Part model, mm, in its own coordinate system. A direction names the side the tool comes from. Round coordinates to 2 decimals unless told otherwise and drop trailing zeros. Loops run counter-clockwise (first coordinate to the right, second up) from the corner with the lowest first, then second, coordinate; pieces in that order, holes last.
1) Probe line 1 (Z direction, x = 14, y = -11); line 2 (Y direction, x = 5.5, z = -8.5); line 3 (X direction, y = -4.5, z = -4.75). List the from-to ranges inside material, lowest first.
2) 3-axis set-ups, long thin cutter, end or side, ignore diameter. For faces 1 (the cylindrical face through (11.48, 1.264, -1.479)), 2 (the flat face through (-13.348, -4, -8)), 3 (the flat face through (8.137, -4, -8)), 4 (the flat face through (15.874, -4, 1)), 5 (the flat face through (12, -2, -3)): which of +Z, -Z, +X, -X, +Y, -Y reach the whole face in a straight line?
3) Band-saw the part on D-D, the plane x = 12.5. Write the cut outline in (y, z).
4) Band-saw the part on C-C, the plane z = 0.5. Write the cut outline in (x, y).
5) Mould opens along Y. For faces 6 (the cylindrical face through (12.621, 4.594, 0.986)), 7 (the cylindrical face through (11.537, -3.02, -1.479)), 8 (the flat face through (-3, 9.656, 1)), 9 (the flat face through (-3, -4, 2)) say: +Y half, -Y half, draft (parallel to the pull), parting line (faces both ways), or undercut.
6) Band-saw the part on B-B, the plane y = 5.25. Write the cut outline in (x, z), then the cut area to 3 significant figures.
7) Band-saw the part on A-A, the plane x = 3.5. Write the cut outline in (y, z), then the cut area to 3 significant figures.
8) Drop flat-ended pins along their axis: P1, Ø3, axis at y = 1, z = -8.5, coming from the +X side; P2, Ø1, axis at x = 12.5, y = -2.5, coming from the -Z side; P3, Ø5, axis at x = -17.53, y = 6.16, coming from the -Z side; P4, Ø1.9, axis at x = -17.53, y = -13.84, coming from the +Z side. Give the stop position or say it passes through.
from build123d import *

# Parameters (mm, degrees)
SKETCH_1_W          = 37
SKETCH_1_H          = 27
EXTRUDE_1_DEPTH     = 2
SKETCH_2_R          = 1.6
CUT_EXTRUDE_1_DEPTH = 28.407139806
SKETCH_3_W          = 21.485092325
SKETCH_3_H          = 12.933183026
EXTRUDE_2_DEPTH     = 17
SKETCH_4_R          = 1
EXTRUDE_3_DEPTH     = 3


with BuildPart() as part:
    # 草圖1 → 填料-伸長1 (new body)
    with BuildSketch(Plane.XY):
        with Locations((-2.626304802, -3.844467641)):
            Rectangle(SKETCH_1_W, SKETCH_1_H)
    extrude(amount=EXTRUDE_1_DEPTH)

    # 草圖2 → 除料-伸長1 (cut, through all)
    with BuildSketch(Plane(origin=(0, 0, 0), x_dir=(-1, 0, 0), z_dir=(0, 0, -1))):
        with Locations((-12.273695198, 6.155532359)):
            Circle(SKETCH_2_R)
        with Locations((-12.273695198, -13.844467641)):
            Circle(SKETCH_2_R)
        with Locations((17.526304802, -13.844467641)):
            Circle(SKETCH_2_R)
        with Locations((17.526304802, 6.155532359)):
            Circle(SKETCH_2_R)
    extrude(amount=-CUT_EXTRUDE_1_DEPTH, mode=Mode.SUBTRACT)

    # 草圖3 → 填料-伸長2 (add)
    with BuildSketch(Plane(origin=(0, 0, 0), x_dir=(-1, 0, 0), z_dir=(0, 0, -1))):
        with Locations((2.605240986, -4.328935409)):
            Rectangle(SKETCH_3_W, SKETCH_3_H)
    extrude(amount=EXTRUDE_2_DEPTH)

    # 草圖4 → 填料-伸長3 (add)
    with BuildSketch(Plane(origin=(0, 0, 0), x_dir=(-1, 0, 0), z_dir=(0, 0, -1))):
        with Locations(Location((-12.273695198, -2.344467641, 0), (0, 0, 180))):
            Circle(SKETCH_4_R)
        with Locations(Location((-12.273695198, -5.344467641, 0), (0, 0, 180))):
            Circle(SKETCH_4_R)
        with Locations(Location((-12.273695198, -8.344467641, 0), (0, 0, 180))):
            Circle(SKETCH_4_R)
        with Locations(Location((-12.273695198, 0.655532359, 0), (0, 0, 180))):
            Circle(SKETCH_4_R)
    extrude(amount=EXTRUDE_3_DEPTH)


solid = part.part
Reported:
1. line 1: z = 0 to 2
1. line 2: y = -10.8 to 2.14
1. line 3: x = -13.35 to 8.14
2. face 1: -Z
2. face 2: -Z, -X, +Y, -Y
2. face 3: -Z, +Y, -Y
2. face 4: +Z, -Z, +X, +Y, -Y
2. face 5: -Z, +X, +Y, -Y
3. outline: (-17.34, 0) - (-15.43, 0) - (-15.43, 2) - (-17.34, 2) - close; (-12.26, 0) - (-9.32, 0) - (-9.32, -3) - (-7.37, -3) - (-7.37, 0) - (-6.32, 0) - (-6.32, -3) - (-4.37, -3) - (-4.37, 0) - (-3.32, 0) - (-3.32, -3) - (-1.37, -3) - (-1.37, 0) - (-0.32, 0) - (-0.32, -3) - (1.63, -3) - (1.63, 0) - (4.57, 0) - (4.57, 2) - (-12.26, 2) - close; (7.74, 0) - (9.66, 0) - (9.66, 2) - (7.74, 2) - close
4. outline: (-21.13, -17.34) - (15.87, -17.34) - (15.87, 9.66) - (-21.13, 9.66) - close; hole circle Ø3.2 at (-17.53, -13.84); hole circle Ø3.2 at (-17.53, 6.16); hole circle Ø3.2 at (12.27, -13.84); hole circle Ø3.2 at (12.27, 6.16)
5. face 6: undercut
5. face 7: undercut
5. face 8: +Y half
5. face 9: draft
6. outline: (-21.13, 0) - (-18.85, 0) - (-18.85, 2) - (-21.13, 2) - close; (-16.21, 0) - (10.95, 0) - (10.95, 2) - (-16.21, 2) - close; (13.59, 0) - (15.87, 0) - (15.87, 2) - (13.59, 2) - close
6. area: 63.4 mm2
7. outline: (-17.34, 0) - (-10.8, 0) - (-10.8, -17) - (2.14, -17) - (2.14, 0) - (9.66, 0) - (9.66, 2) - (-17.34, 2) - close
7. area: 274 mm2
8. P1: stops at x = 8.14
8. P2: stops at z = -3
8. P3: stops at z = 0
8. P4: passes through
